from build123d import *

# Parameters (mm, degrees)
SKETCH2_R           = 6.35
BOSS_EXTRUDE1_DEPTH = 7.9375
SKETCH7_R           = 19
BOSS_EXTRUDE5_DEPTH = 18
SKETCH8_R           = 1.7
CUT_EXTRUDE1_DEPTH  = 39.524506895
SKETCH9_R           = 2.8
CUT_EXTRUDE2_DEPTH  = 3.4
SKETCH6_R           = 2.2
CUT_EXTRUDE3_DEPTH  = 39.524506895
SKETCH10_R          = 3.9
CUT_EXTRUDE4_DEPTH  = 3
BOSS_EXTRUDE6_DEPTH = 1.5
SKETCH11_R          = 0.8
BOSS_EXTRUDE7_DEPTH = 3
SKETCH12_R          = 6
CUT_EXTRUDE5_DEPTH  = 10


with BuildPart() as part:
    # Sketch2 → Boss-Extrude1 (new body)
    with BuildSketch(Plane(origin=(0, 0, 0), x_dir=(1, 0, 0), z_dir=(0, 1, 0))):
        with Locations(Location((0, 0, 0), (0, 0, 270))):
            Circle(SKETCH2_R)
    extrude(amount=BOSS_EXTRUDE1_DEPTH)

    # Sketch7 → Boss-Extrude5 (add)
    with BuildSketch(Plane.XZ):
        with Locations(Location((2.222246, 0, 0), (0, 0, 270))):
            Circle(SKETCH7_R)
    extrude(amount=BOSS_EXTRUDE5_DEPTH)

    # Sketch8 → Cut-Extrude1 (cut, through all)
    with BuildSketch(Plane.XZ.offset(18)):
        with Locations(Location((2.222246, 15.5, 0), (0, 0, 270))):
            Circle(SKETCH8_R)
        with Locations(Location((17.722246, 0, 0), (0, 0, 270))):
            Circle(SKETCH8_R)
        with Locations(Location((2.222246, -15.5, 0), (0, 0, 270))):
            Circle(SKETCH8_R)
        with Locations(Location((-13.277754, 0, 0), (0, 0, 270))):
            Circle(SKETCH8_R)
    extrude(amount=-CUT_EXTRUDE1_DEPTH, mode=Mode.SUBTRACT)

    # Sketch9 → Cut-Extrude2 (cut)
    with BuildSketch(Plane(origin=(0, 0, 0), x_dir=(1, 0, 0), z_dir=(0, 1, 0))):
        with Locations(Location((2.222246, 15.5, 0), (0, 0, 270))):
            Circle(SKETCH9_R)
        with Locations(Location((17.722246, 0, 0), (0, 0, 270))):
            Circle(SKETCH9_R)
        with Locations(Location((2.222246, -15.5, 0), (0, 0, 270))):
            Circle(SKETCH9_R)
        with Locations(Location((-13.277754, 0, 0), (0, 0, 270))):
            Circle(SKETCH9_R)
    extrude(amount=-CUT_EXTRUDE2_DEPTH, mode=Mode.SUBTRACT)

    # Sketch6 → Cut-Extrude3 (cut, through all)
    with BuildSketch(Plane(origin=(0, 7.9375, 0), x_dir=(1, 0, 0), z_dir=(0, 1, 0))):
        with Locations(Location((0.952246, 0, 0), (0, 0, 270))):
            Circle(SKETCH6_R)
    extrude(amount=-CUT_EXTRUDE3_DEPTH, mode=Mode.SUBTRACT)

    # Sketch10 → Cut-Extrude4 (cut)
    with BuildSketch(Plane.XZ.offset(18)):
        with Locations(Location((0.952246, 0, 0), (0, 0, 270))):
            Circle(SKETCH10_R)
    extrude(amount=-CUT_EXTRUDE4_DEPTH, mode=Mode.SUBTRACT)

    # Sketch4 → Boss-Extrude6 (add)
    with BuildSketch(Plane(origin=(0, 7.9375, 0), x_dir=(1, 0, 0), z_dir=(0, 1, 0))):
        with BuildLine():
            ThreePointArc((2.221123, 5.948874904), (-1.907754, 0), (2.221123, -5.948874904))
            ThreePointArc((2.221123, -5.948874904), (-6.35, 0), (2.221123, 5.948874904))
        make_face()
    extrude(amount=BOSS_EXTRUDE6_DEPTH)

    # Sketch11 → Boss-Extrude7 (add)
    with BuildSketch(Plane(origin=(0, 7.9375, 0), x_dir=(1, 0, 0), z_dir=(0, 1, 0))):
        with Locations(Location((0.952246, 3.8, 0), (0, 0, 270))):
            Circle(SKETCH11_R)
        with Locations(Location((0.952246, -3.8, 0), (0, 0, 270))):
            Circle(SKETCH11_R)
    extrude(amount=BOSS_EXTRUDE7_DEPTH)

    # Sketch12 → Cut-Extrude5 (cut)
    with BuildSketch(Plane.XZ.offset(18)):
        with Locations(Location((2.222246, 0, 0), (0, 0, 270))):
            Circle(SKETCH12_R)
    extrude(amount=-CUT_EXTRUDE5_DEPTH, mode=Mode.SUBTRACT)


solid = part.part
The listing builds one solid part. Answer for the finished solid, in the listing's coordinates (mm). A direction names the side the tool comes from. Round coordinates to 2 decimals unless told otherwise and drop trailing zeros. Loops run counter-clockwise (first coordinate to the right, second up) from the corner with the lowest first, then second, coordinate; pieces in that order, holes last. Notation, with made-up numbers: M 57.25,-19 L 100.25,-19 A10 ccw 100.25,-6 Z; hole C -35,45 d3. An arc over 180 degrees is marked long. Return JSON: item names as keys, results as strings.
Q1. Each of these flat-tipped pins is pushed along its axis until it touches: pin 1 Ø3 at (x, z) = (2.22, -15.5) entering from +Y; pin 2 Ø6 at (x, z) = (17, -1) entering from +Y; pin 3 Ø4 at (x, y) = (-0.5, 4) entering from -Z; pin 4 Ø3 at (x, z) = (2.5, -15.5) entering from +Y. Where does it stop, or does it pass through?
Results list:
{"pin 1": "passes through", "pin 2": "stops at y = 0", "pin 3": "stops at z = -6.35", "pin 4": "stops at y = -3.4"}
Q2. Find section A-A, the plane z = 0. State how many separate pieces and enclosed holes the cut face has, plus the area to 3 significant figures.
Results list:
{"separate pieces": "4", "enclosed holes": "0", "area": "464 mm2"}
Q3. Find the intervals of material crossed by line 1 along X through (y, z) = (-11, 0); line 2 along Z through (x, y) = (1.5, -14.25); line 3 along Z through (x, y) = (-13, -13.5), in increasing order. Write a range as from..to.
Results list:
{"line 1": "x = -16.78..-14.98, -11.58..-3.78, 8.22..16.02, 19.42..21.22", "line 2": "z = -18.99..-17.04, -13.96..-5.96, 5.96..13.96, 17.04..18.99", "line 3": "z = -11.37..-1.68, 1.68..11.37"}
Q4. Find section B-B, the plane z = -15.5. Determine the outline of the cut face in (x, y).
Results list:
{"outline": "M -8.77,-18 L 0.52,-18 L 0.52,-3.4 L -0.58,-3.4 L -0.58,0 L -8.77,0 Z; M 3.92,-18 L 13.21,-18 L 13.21,0 L 5.02,0 L 5.02,-3.4 L 3.92,-3.4 Z"}
Q5. Find section C-C, the plane x = 15.5. Determine the outline of the cut face in (y, z), plus the area to 3 significant figures.
Results list:
{"outline": "M -18,-13.59 L 0,-13.59 L 0,-1.7 L -3.4,-1.7 L -3.4,1.7 L 0,1.7 L 0,13.59 L -18,13.59 Z", "area": "478 mm2"}
Q6. Find section D-D, the plane y = -6.25. Determine the outline of the cut face in (x, z).
Results list:
{"outline": "C 2.22,0 d38; hole C -13.28,0 d3.4; hole C 0.95,0 d4.4; hole C 2.22,-15.5 d3.4; hole C 2.22,15.5 d3.4; hole C 17.72,0 d3.4"}
Q7. Which of the six approach directions +Z, -Z, +X, -X, +Y, -Y give full straight-line access (tool end or side, diameter ignored) to faces 4 (the face through (-14.937, -10.802, 0.369)), 5 (the face through (20.08, -1.68, 1.51))?
Results list:
{"face 4": "+Y, -Y", "face 5": "+Y"}
Q8. The mould has two halves that part along X. Classify faces 1 (the face through (1, 10.938, 4)), 2 (the face through (4.024, -13.07, -5.723)), 3 (the face through (-16.326, -8.874, 4.119)): released by +X, released by -X, zero draft, split by the parting line, or undercut.
Results list:
{"face 1": "zero draft", "face 2": "undercut", "face 3": "split by the parting line"}
